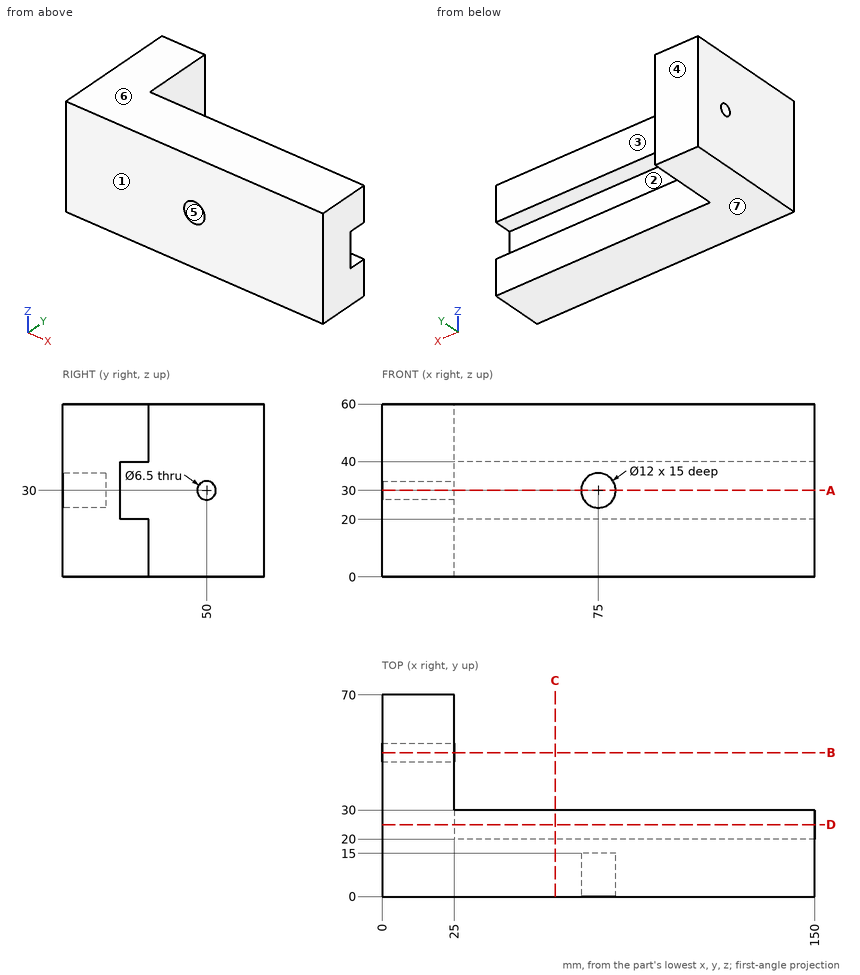
For this review, use the dimensioned drawing (mm, ordinates from the lowest corner) and the shaded views. A direction names the side the tool comes from. Round coordinates to 2 decimals unless told otherwise and drop trailing zeros. Order: outer loops, then holes, each group sorted by start corner. A loop starts at its lowest first (then second) coordinate and runs counter-clockwise, first axis right, second up. Notation, with made-up numbers: (1, -24) -> (8, -24) arc R18 cw to (8, -2) -> close; hole circle Ø5 at (39, -0.75). An arc over 180 degrees is marked (long way). One line per item, written item: value. Start each with the question number.
Q1. Mouldability with a two-part tool opening along Z and no side actions: class the marked faces 4, 5, 6 and 7 as released by +Z, released by -Z, zero draft, split by the parting line, or undercut.
Q2. Machinability: for the marked faces 1, 2 and 3, which of the approach directions +Z, -Z, +X, -X, +Y, -Y give a long, thin tool a straight path to every point of the face, cutting with its end or side? Answer none if there is none.
Q3. Take a section at D-D (y = 25). Write out the cut boundary in (x, z).
Q4. Take a section at B-B (y = 50). Write out the cut boundary in (x, z), and give its area (3 significant figures).
Q5. Take a section at A-A (z = 30). Write out the cut boundary in (x, y), and give its area (3 significant figures).
Q6. Take a section at C-C (x = 60). Write out the cut boundary in (y, z), and give its area (3 significant figures).
Q7. Clearance check with flat-ended pins moving along their axes: pin 1 Ø12 at (x, z) = (93.5, 16) entering from +Y; pin 2 Ø6 at (y, z) = (50, 30) entering from -X; pin 3 Ø1 at (y, z) = (42.5, 11.5) entering from +X. State where each tip first meets the part, or that it passes through.
Q8. Wall thickness on line 1 (Z direction, x = 75, y = 10.5); line 2 (Y direction, x = 6.5, z = 30); line 3 (Y direction, x = 69.5, z = 56.5): over which ranges is each line inside the solid? List them lowest first.
Reported:
1. face 4: zero draft
1. face 5: undercut
1. face 6: released by +Z
1. face 7: released by -Z
2. face 1: +Z, -Z, +X, -X, -Y
2. face 2: +X, +Y
2. face 3: +Z, -Z, +X, +Y
3. outline: (0, 0) -> (150, 0) -> (150, 20) -> (25, 20) -> (25, 40) -> (150, 40) -> (150, 60) -> (0, 60) -> close
4. outline: (0, 0) -> (25, 0) -> (25, 26.75) -> (0, 26.75) -> close; (0, 33.25) -> (25, 33.25) -> (25, 60) -> (0, 60) -> close
4. area: 1,340 mm2
5. outline: (0, 0) -> (69, 0) -> (69, 15) -> (81, 15) -> (81, 0) -> (150, 0) -> (150, 20) -> (25, 20) -> (25, 46.75) -> (0, 46.75) -> close; (0, 53.25) -> (25, 53.25) -> (25, 70) -> (0, 70) -> close
5. area: 3,910 mm2
6. outline: (0, 0) -> (30, 0) -> (30, 20) -> (20, 20) -> (20, 40) -> (30, 40) -> (30, 60) -> (0, 60) -> close
6. area: 1,600 mm2
7. pin 1: stops at y = 30
7. pin 2: passes through
7. pin 3: stops at x = 25
8. line 1: z = 0 to 24, 36 to 60
8. line 2: y = 0 to 46.75, 53.25 to 70
8. line 3: y = 0 to 30
